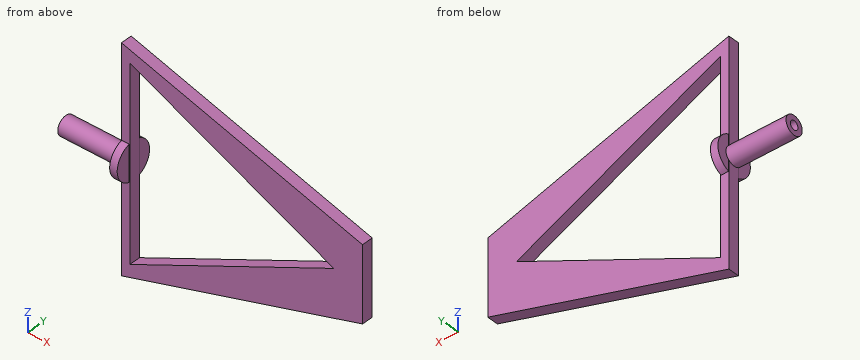
Autodesk Inventor part; units mm, degrees
ref_plane "YZ Plane" through (0, 0, 0) normal (1, 0, 0) x (0, 1, 0)
ref_plane "XY Plane" through (0, 0, 0) normal (0, 0, 1) x (1, 0, 0)
sketch "Sketch1" plane through (0, 0, 0) normal (0, 1, 0) x (-1, 0, 0)
  arc A0 (0, -5) -> (0, 5) centre (0, 0) ccw
  line L0 (0, 5) -> (0, -5)
  dimension "d0" = 10
extrude "Extrusion1" add sketch "Sketch1" along normal blind 10
sketch "Sketch2" plane through (0, 0, 0) normal (1, 0, 0) x (0, 1, 0)
  line L0 (8.0172, -4.5) -> (8.0172, 4.5)
  line L1 (8.0172, 4.5) -> (2.5172, 4.5)
  line L2 (2.5172, -4.5) -> (0.0172, -2)
  line L3 (2.5172, 4.5) -> (0.0172, 2)
  line L4 (0.0172, -2) -> (0.0172, 2)
  line L5 (8.0172, -4.5) -> (2.5172, -4.5)
  point P0 (0, 0)
  dimension "d3" = 9
  dimension "d4" = 8
sketch "Sketch3" plane through (0, 0, 0) normal (1, 0, 0) x (0, 1, 0)
  line L0 (0, 2) -> (3, 5)
  arc A0 (3, 5) -> (0, 2) centre (1, 4) ccw
  line L1 (0, -2) -> (4, -6)
  arc A1 (0, -2) -> (4, -6) centre (1.75, -4.25) ccw
  line L2 (8.0325, 5) -> (11, 5)
  line L3 (11, 5) -> (11, -6)
  line L4 (11, -6) -> (8.0325, -6)
  line L5 (8.0325, -6) -> (8.0325, 5)
  line L6 (2.4911, 4.4911) -> (5, 7)
  line L7 (2.4911, 4.4911) -> (8.0325, 4.4911)
  arc A2 (8.0325, 4.4911) -> (5, 7) centre (7, 6.3303) ccw
  line L8 (2.4911, -4.4911) -> (8.5706, -4.4911)
  arc A3 (2.4911, -4.4911) -> (8.5706, -4.4911) centre (5.5309, -7.5041) ccw
  point P0 (0, 0)
extrude "Extrusion2" cut sketch "Sketch3" against normal through all
sketch "Sketch4" plane through (0, 0, 0) normal (0, 1, 0) x (-1, 0, 0)
  arc A0 (1.0726, -4.4911) -> (1.0726, 4.4911) centre (-1.125, 0) ccw
  arc A1 (1.0726, 4.4911) -> (1.0726, -4.4911) centre (-0.4517, 0) ccw
  point P0 (0, 0)
  point P1 (2.1976, -4.4911)
  point P2 (2.1976, 4.4911)
  dimension "d9" = 1.125
  dimension "d10" = 1.125
extrude "Extrusion3" cut sketch "Sketch4" along normal through all both and the other way through all
sketch "Sketch5" plane through (0, 0, 0) normal (1, 0, 0) x (0, 1, 0)
  line L0 (1.6, -1.2445) -> (1.6, 1.1555)
  line L1 (6.4325, 2.6911) -> (3.1125, 2.6911)
  line L2 (6.4325, -2.6911) -> (6.4325, 2.6911)
  line L3 (6.4325, -2.6911) -> (3.1125, -2.6911)
  line L4 (0, 2) -> (0, -2)
  line L5 (8.0325, 4.4911) -> (8.0325, -4.4911)
  line L6 (0, 2) -> (2.4911, 4.4911)
  line L7 (2.4911, 4.4911) -> (8.0325, 4.4911)
  line L8 (8.0325, 4.4911) -> (8.0325, -4.4911)
  line L9 (8.0325, -4.4911) -> (2.4911, -4.4911)
  line L10 (2.4911, -4.4911) -> (0, -2)
  line L11 (0, 2) -> (0, -2)
  line L12 (1.6, 1.1555) -> (3.1125, 2.6911)
  line L13 (1.6, -1.2445) -> (3.1125, -2.6911)
  line L14 (1.6, 4.6579) -> (1.6, -5.3823)
  arc A0 (1.6, 4.6579) -> (1.6, -5.3823) centre (3.2437, -0.3622) ccw
  line L15 (1.6, 1.1555) -> (5.4757, 5.0906)
  line L16 (1.6, 1.1555) -> (1.6, 7.5999)
  arc A1 (5.4757, 5.0906) -> (1.6, 7.5999) centre (3.8837, 6.8794) ccw
  line L17 (3.1125, 2.6911) -> (12.4034, 2.6911)
  line L18 (3.1125, 2.6911) -> (8.5318, 8.1936)
  arc A2 (12.4034, 2.6911) -> (8.5318, 8.1936) centre (8.3272, 3.9364) ccw
  line L19 (6.4325, 2.6911) -> (13.6333, 2.6911)
  line L20 (6.4325, 2.6911) -> (6.4325, -9.3636)
  arc A3 (6.4325, -9.3636) -> (13.6333, 2.6911) centre (6.37, -1.1482) ccw
  line L21 (6.4325, -2.6911) -> (6.4325, -11.5775)
  line L22 (6.4325, -2.6911) -> (3.1125, -2.6911)
  line L23 (3.1125, -2.6911) -> (3.2437, -12.8567)
  arc A4 (3.2437, -12.8567) -> (6.4325, -9.3636) centre (5.6123, -11.8169) ccw
  line L24 (1.6, -1.2445) -> (1.6, -8.2222)
  line L25 (1.6, -1.2445) -> (3.1125, -2.6911)
  line L26 (3.1125, -2.6911) -> (3.1946, -9.0574)
  arc A5 (1.6, -8.2222) -> (3.1946, -9.0574) centre (2.6381, -8.1801) ccw
  point P0 (0, 0)
  dimension "d16" = 1.6
  dimension "d18" = 1.6
  dimension "d21" = 1.8
  dimension "d23" = 1.8
  dimension "d24" = 2.4
  dimension "d26" = 3.32
  dimension "d27" = 3.32
extrude "Extrusion4" cut sketch "Sketch5" against normal through all contours L14 L10 L4 L6 L0 | L13 L23 L9 L10 L14 | L14 L6 L7 L15 L12 | L3 L20 L9 L23 | L14 A0 L6 L4 L10 | L10 L9 L23 A5 L24 L14 | L15 L7 L5 L17 L1 | L14 L16 A1 L15 L7 L6 | L2 L17 L5 L9 L20 | L9 L20 A4 L23 | L15 L18 A2 L17 L5 L7 | L9 L5 L17 L19 A3 L20
sketch "Sketch6" plane through (0, 0, 0) normal (1, 0, 0) x (0, 1, 0)
  circle A0 centre (4, 0) radius 2.5
  line L0 (1.6, -1.2445) -> (1.6, 1.1555)
  point P0 (0, 0)
  dimension "d31" = 5
  dimension "d32" = 2.4
extrude "Extrusion5" add sketch "Sketch6" against normal blind 15
sketch "Sketch7" plane through (0, 0, 0) normal (0, 1, 0) x (-1, 0, 0)
  arc A0 (3.089, -2.6911) -> (3.7176, -1.2445) centre (-1.125, 0) ccw
  arc A1 (3.7397, 1.1555) -> (3.089, 2.6911) centre (-1.125, 0) ccw
  arc A2 (3.7176, -1.2445) -> (3.7397, 1.1555) centre (-1.125, 0) ccw
  arc A3 (3.089, 2.6911) -> (3.089, -2.6911) centre (1.3425, 0) ccw
  point P0 (0, 0)
extrude "Extrusion6" cut sketch "Sketch7" along normal through all
sketch "Sketch8" plane through (-15, 4, 0) normal (-1, 0, 0) x (0, 0, 1)
  circle A0 centre (0, 0) radius 0.5875
  point P0 (0, -4)
  dimension "d37" = 1.175
extrude "Extrusion7" cut sketch "Sketch8" against normal blind 7
sketch "Sketch9" plane through (0, 0, 0) normal (0, 1, 0) x (-1, 0, 0)
  line L0 (6, 3) -> (2, 3)
  line L1 (2, 3) -> (2, -3)
  line L2 (2, -3) -> (6, -3)
  line L3 (6, -3) -> (6, 3)
  point P0 (0, 0)
extrude "Extrusion8" cut sketch "Sketch9" along normal through all both and the other way through all
sketch "Sketch10" plane through (-15, 4, 0) normal (-1, 0, 0) x (0, 0, 1)
  circle A0 centre (0, 0) radius 1.25
  circle A1 centre (0, 0) radius 3.9528
  point P0 (0, -4)
  dimension "d69" = 2.5
extrude "Extrusion9" cut sketch "Sketch10" against normal blind 8
ref_plane "Work Plane1" through (0, 4.1, 0) normal (0, 1, 0) x (-1, 0, 0)
sketch "Sketch12" plane through (0, 4.1, 0) normal (0, 1, 0) x (-1, 0, 0)
  line L0 (15, -1) -> (15, 1)
  line L1 (5.9113, 12.6879) -> (5.9113, -12.7121)
  line L2 (5.9113, 12.6879) -> (-21.266, 0.1332)
  line L3 (-21.266, 0.1332) -> (5.9113, -12.7121)
  line L4 (7.0341, 14.6962) -> (7.0341, -14.7038)
  line L5 (2.03, -0.0038) -> (19.03, -0.0038)
  line L6 (-25.0887, 5) -> (-25.0887, -5)
  line L7 (-25.0887, 5) -> (7.0341, 14.6962)
  line L8 (-25.0887, -5) -> (7.0341, -14.7038)
  point P0 (0, 0)
  point P1 (0, 0)
  dimension "d61" = 25.4
  dimension "d62" = 29.4
  dimension "d63" = 14.7
  dimension "d64" = 10
  dimension "d67" = 31
extrude "Extrusion11" add sketch "Sketch12" along normal mid plane 1.5
properties part number "piezo_mounted_whisk_deflector_SHORT"
Read the model definition and answer for the solid it produces. Units are mm, in the model's axes. Round coordinates to 2 decimals unless told otherwise and drop trailing zeros. Write each loop counter-clockwise with the first axis right and the second up, starting at its lowest first coordinate (ties: lowest second). Pieces come first, ordered by that corner, then holes.
1. The part is cut by section C-C, the plane y = 4. Determine the outline of the cut face in (x, z), then the cut area to 3 significant figures.
2. The part is cut by section B-B, the plane x = 3. Determine the outline of the cut face in (y, z), then the cut area to 3 significant figures.
3. The part is cut by section A-A, the plane z = 3.75. Determine the outline of the cut face in (x, y), then the cut area to 3 significant figures.
4. Straight lines are drawn through the part: L1, parallel to Y at x = -12.25, z = 0; L2, parallel to Y at x = -6, z = 9.25; L3, parallel to Y at x = -11, z = 0.25. For each, find the intervals that lie inside material, in ascending order.
5. Given pin 1 Ø0.5 at (y, z) = (4.5, -11) entering from -X; pin 2 Ø1.3 at (y, z) = (6, 0.5) entering from +X; pin 3 Ø3 at (x, y) = (-5.5, 2.5) entering from -Z; pin 4 Ø2 at (x, z) = (-9.5, -11.5) entering from +Y, each flat-ended and moving along its own axis, determine where each tip first touches the part or whether it passes through.
6. The part is cut by section D-D, the plane x = 22. Determine the outline of the cut face in (y, z).
Values:
1. outline: (-15, -1.25) - (-7.03, -1.25) - (-7.03, -14.7) - (25.09, -5) - (25.09, 5) - (-7.03, 14.7) - (-7.03, 1.25) - (-15, 1.25) - (-15, 0.59) - (-8, 0.59) - (-8, -0.59) - (-15, -0.59) - close; hole (-5.91, -12.71) - (21.27, 0.13) - (-5.91, 12.69) - close
1. area: 299 mm2
2. outline: (3.35, -11.67) - (4.85, -11.67) - (4.85, -8.5) - (3.35, -8.5) - close; (3.35, 8.57) - (4.85, 8.57) - (4.85, 11.67) - (3.35, 11.67) - close
2. area: 9.40 mm2
3. outline: (-7.03, 3.35) - (-5.91, 3.35) - (-5.91, 4.85) - (-7.03, 4.85) - close; (13.44, 3.35) - (25.09, 3.35) - (25.09, 4.85) - (13.44, 4.85) - close
3. area: 19.2 mm2
4. L1: y = 2.75 to 3.41, 4.59 to 5.25
4. L2: y = 3.35 to 4.85
4. L3: y = 2.78 to 3.47, 4.53 to 5.22
5. pin 1: stops at x = -7.03
5. pin 2: stops at x = -6
5. pin 3: stops at z = -14.61
5. pin 4: passes through
6. outline: (3.35, -5.93) - (4.85, -5.93) - (4.85, 5.93) - (3.35, 5.93) - close
